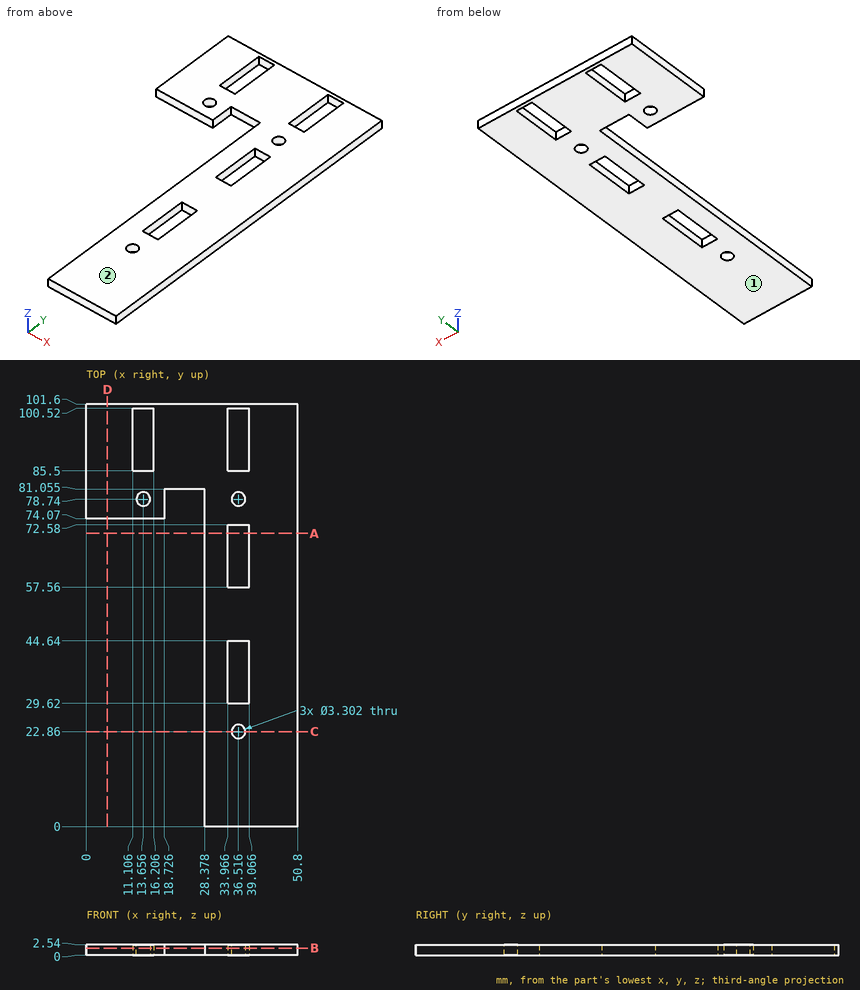
Study the drawing (mm; zero at the part's minimum x, y, z) and answer. Give positions to 0.01 mm unless a question says otherwise; leave off trailing zeros. Loops run counter-clockwise (first coordinate to the right, second up) from the corner with the lowest first, then second, coordinate; pieces in that order, holes last. Notation, with made-up numbers: (28.25, 68) - (65.25, 68) arc R36 ccw to (65.25, 105) - close; hole circle Ø6 at (77.5, 10). An arc over 180 degrees is marked (long way). Answer in a Markdown table with one row per item. Add a question column.
Q1. Determine the mould class of the marked faces 1 and 2 for opening direction Z: released by +Z, released by -Z, zero draft, split by the parting line, or undercut.
Q2. Consider line 1 along X through (y, z) = (78.74, 1.25) (3 decimals); line 2 along X through (y, z) = (90.5, 0.2); line 3 along Y through (x, z) = (36, 1.4). Determine where each line is inside the solid, lowest interval first.
Q3. The part is cut by section B-B (z = 1.7). Determine the outline of the cut face in (x, y) (3 decimals).
Q4. The part is cut by section A-A (y = 70.5). Determine the outline of the cut face in (x, z).
Q5. Each of these flat-tipped pins is pushed along its axis until it touches: P1, Ø0.8, axis at x = 9, z = 1.5, coming from the -Y side; P2, Ø0.8, axis at y = 53.5, z = 1, coming from the -X side. Where does it stop, or does it pass through?
Q6. The part is cut by section C-C (y = 22.86). Determine the outline of the cut face in (x, z) (3 decimals), and give its area (3 significant figures).
Q7. The part is cut by section D-D (x = 5). Determine the outline of the cut face in (y, z).
Solution:
| question | item | result |
|---|---|---|
| 1 | face 1 | released by -Z |
| 1 | face 2 | released by +Z |
| 2 | line 1 | x = 0 to 12.005, 15.307 to 18.726, 28.378 to 34.865, 38.167 to 50.8 |
| 2 | line 2 | x = 0 to 11.11, 16.21 to 33.97, 39.07 to 50.8 |
| 2 | line 3 | y = 0 to 21.29, 24.43 to 29.62, 44.64 to 57.56, 72.58 to 77.17, 80.31 to 85.5, 100.52 to 101.6 |
| 3 | outline | (0, 74.07) - (18.726, 74.07) - (18.726, 81.055) - (28.378, 81.055) - (28.378, 0) - (50.8, 0) - (50.8, 101.6) - (0, 101.6) - close; hole (11.106, 85.5) - (16.206, 85.5) - (16.206, 100.52) - (11.106, 100.52) - close; hole circle Ø3.302 at (13.656, 78.74); hole (33.966, 29.62) - (39.066, 29.62) - (39.066, 44.64) - (33.966, 44.64) - close; hole (33.966, 57.56) - (39.066, 57.56) - (39.066, 72.58) - (33.966, 72.58) - close; hole (33.966, 85.5) - (39.066, 85.5) - (39.066, 100.52) - (33.966, 100.52) - close; hole circle Ø3.302 at (36.516, 22.86); hole circle Ø3.302 at (36.516, 78.74) |
| 4 | outline | (28.38, 0) - (33.97, 0) - (33.97, 2.54) - (28.38, 2.54) - close; (39.07, 0) - (50.8, 0) - (50.8, 2.54) - (39.07, 2.54) - close |
| 5 | P1 | stops at y = 74.07 |
| 5 | P2 | stops at x = 28.38 |
| 6 | outline | (28.378, 0) - (34.865, 0) - (34.865, 2.54) - (28.378, 2.54) - close; (38.167, 0) - (50.8, 0) - (50.8, 2.54) - (38.167, 2.54) - close |
| 6 | area | 48.6 mm² |
| 7 | outline | (74.07, 0) - (101.6, 0) - (101.6, 2.54) - (74.07, 2.54) - close |
